from build123d import *

# Parameters (mm, degrees)
SKETCH1_W               = 200
SKETCH1_H               = 240
BOSS_EXTRUDE1_DEPTH     = 20
SKETCH2_W               = 200
SKETCH2_H               = 40
BOSS_EXTRUDE2_DEPTH     = 110
SKETCH3_W               = 200
SKETCH3_H               = 40
BOSS_EXTRUDE3_DEPTH     = 110
RIB1_REACH              = 205.224
SKETCH4_WALL_W          = 636.702272868
SKETCH4_WALL_H          = 40
RIB2_REACH              = 205.224
SKETCH6_WALL_W          = 636.702272868
SKETCH6_WALL_H          = 40
CUT_EXTRUDE1_DEPTH      = 259.650343128
CUT_EXTRUDE1_DEPTH_BACK = 259.650343128
SKETCH7_R               = 24


with BuildPart() as part:
    # Sketch1 → Boss-Extrude1 (new, symmetric)
    with BuildSketch(Plane.YZ):
        Rectangle(SKETCH1_W, SKETCH1_H)
    extrude(amount=BOSS_EXTRUDE1_DEPTH, both=True)

    # Sketch2 → Boss-Extrude2 (add)
    with BuildSketch(Plane.YZ.offset(20)):
        with Locations((0, 100)):
            Rectangle(SKETCH2_W, SKETCH2_H)
    extrude(amount=BOSS_EXTRUDE2_DEPTH)

    # Sketch3 → Boss-Extrude3 (add)
    with BuildSketch(Plane(origin=(-20, 0, 0), x_dir=(0, -1, 0), z_dir=(-1, 0, 0))):
        with Locations((0, -100)):
            Rectangle(SKETCH3_W, SKETCH3_H)
    extrude(amount=BOSS_EXTRUDE3_DEPTH)

    # Sketch4 wall → Rib1 (add, up to next)
    with BuildSketch(Plane(origin=(75, 0, -20), x_dir=(-0.481918749772, 0, -0.876215908677), z_dir=(-0.876215908677, 0, 0.481918749772)), mode=Mode.PRIVATE) as rib1_sk1:
        Rectangle(SKETCH4_WALL_W, SKETCH4_WALL_H)
    rib1_tool1 = extrude(rib1_sk1.sketch, amount=RIB1_REACH, mode=Mode.PRIVATE) - part.part
    add(rib1_tool1.solids().sort_by_distance((75, 0, -20))[0])

    # Sketch6 wall → Rib2 (add, up to next)
    with BuildSketch(Plane(origin=(-75, 0, 20), x_dir=(-0.481918749772, 0, -0.876215908677), z_dir=(-0.876215908677, 0, 0.481918749772)), mode=Mode.PRIVATE) as rib2_sk1:
        Rectangle(SKETCH6_WALL_W, SKETCH6_WALL_H)
    rib2_tool1 = extrude(rib2_sk1.sketch, amount=-RIB2_REACH, mode=Mode.PRIVATE) - part.part
    add(rib2_tool1.solids().sort_by_distance((-75, 0, 20))[0])

    # Sketch7 → Cut-Extrude1 (cut, two sides: drawn at the far end of the back side and taken through both)
    with BuildSketch(Plane.XY.offset(-80).offset(-CUT_EXTRUDE1_DEPTH_BACK)):
        with Locations((-82, -60)):
            Circle(SKETCH7_R)
        with Locations(Location((-82, 60, 0), (0, 0, 180))):
            Circle(SKETCH7_R)
    extrude(amount=CUT_EXTRUDE1_DEPTH + CUT_EXTRUDE1_DEPTH_BACK, mode=Mode.SUBTRACT)


solid = part.part
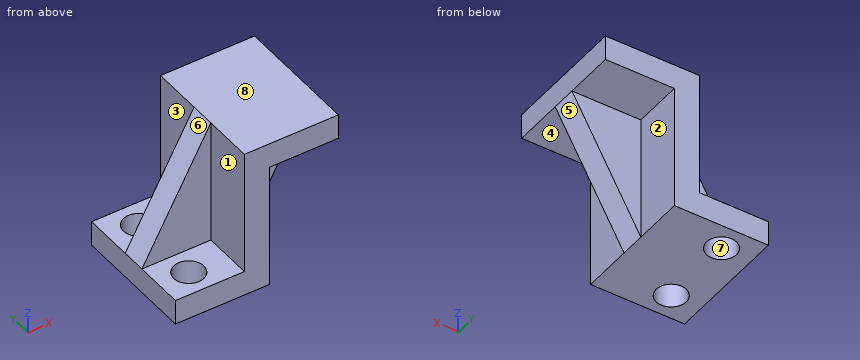
Design review of the part built by this model. Coordinates are the model's own, in mm. Face numbers are marked on the shaded views. A direction names the side the tool comes from. Coordinates: 2 decimals unless noted, no trailing zeros. Order: outer loops, then holes, each group sorted by start corner. A loop starts at its lowest first (then second) coordinate and runs counter-clockwise, first axis right, second up. Notation, with made-up numbers: (3, 4) - (11, 4) arc R33 cw to (11, 33) - close; hole circle Ø5 at (-32.5, 45.25). An arc over 180 degrees is marked (long way). Put each result on its own line as item: value.
1) Wall thickness on L1, parallel to Y at x = -82, z = -108; L2, parallel to X at y = -60, z = -98; L3, parallel to Y at x = 75, z = 53.5: over which ranges is each line inside the solid? List them lowest first. Write a range as from..to.
Response values:
L1: y = -100..-84, -36..36, 84..100
L2: x = -130..-106, -58..20
L3: y = -20..20
2) Insertion check: P1, Ø6, axis at x = 93.5, y = 30, coming from the -Z side; P2, Ø6, axis at y = 62.5, z = -16, coming from the +X side; P3, Ø24, axis at y = 53.5, z = -2.5, coming from the -X side. Each pin has a flat end and moves straight along its axis. Give the tip position at first contact, or say it passes through.
Response values:
P1: stops at z = 80
P2: stops at x = 20
P3: stops at x = -20
3) Take a section at D-D, the plane x = -64. Give the boundary of the cut face in (y, z).
Response values:
outline: (-100, -120) - (-75.87, -120) - (-75.87, -80) - (-100, -80) - close; (-44.13, -120) - (44.13, -120) - (44.13, -80) - (20, -80) - (20, 40) - (-20, 40) - (-20, -80) - (-44.13, -80) - close; (75.87, -120) - (100, -120) - (100, -80) - (75.87, -80) - close
4) Take a section at B-B, the plane z = 100. Give the boundary of the cut face in (x, y), and give its area (3 significant figures).
Response values:
outline: (-31, -20) - (-20, -20) - (-20, -100) - (130, -100) - (130, 100) - (-20, 100) - (-20, 20) - (-31, 20) - close
area: 30,400 mm²
5) Take a section at C-C, the plane y = -23.5. Give the boundary of the cut face in (x, z), and give its area (3 significant figures).
Response values:
outline: (-130, -120) - (20, -120) - (20, 80) - (130, 80) - (130, 120) - (-20, 120) - (-20, -80) - (-130, -80) - close
area: 18,400 mm²
6) Tool access review of the marked faces 1, 2, 3 and 4: name each direction out of +Z, -Z, +X, -X, +Y, -Y from which nothing blocks a thin tool from reaching the whole face with its end or side.
Response values:
face 1: +Z, -X, -Y
face 2: -Z, +X, +Y
face 3: +Z, -X, +Y
face 4: -Z, +X, -Y
7) The part is to be moulded in two halves that separate along X. For the marked faces 5, 6, 7 and 8, say which applies: released by +X, released by -X, zero draft, split by the parting line, or undercut.
Response values:
face 5: released by +X
face 6: released by -X
face 7: undercut
face 8: zero draft
8) Take a section at A-A, the plane y = -60. Give the boundary of the cut face in (x, z).
Response values:
outline: (-130, -120) - (-106, -120) - (-106, -80) - (-130, -80) - close; (-58, -120) - (20, -120) - (20, 80) - (130, 80) - (130, 120) - (-20, 120) - (-20, -80) - (-58, -80) - close
